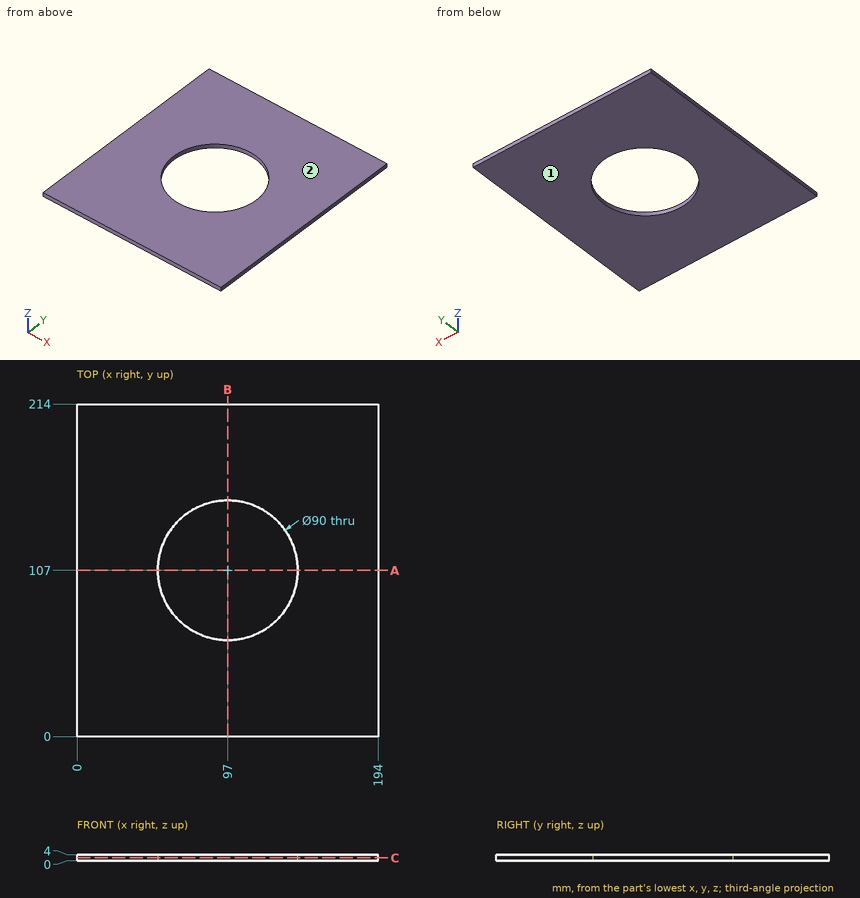
Can you work these out from the drawing? Everything is in mm from the part's minimum corner. Coordinates: 2 decimals unless noted, no trailing zeros. Order: outer loops, then holes, each group sorted by start corner. A loop starts at its lowest first (then second) coordinate and runs counter-clockwise, first axis right, second up. Notation, with made-up numbers: M -6.75,34.5 L 26.25,34.5 A9 ccw 26.25,46.5 Z; hole C 66.25,-26.5 d6. An arc over 180 degrees is marked long. Answer as CSV lines item,"result". Start each with the question number.
1. I want a section at B-B, the plane x = 97. Write out the boundary of the cut face in (y, z), and give its area (3 significant figures).
2. For pin 1 (6 mm diameter, centred on x = 108.5, y = 69.5, fed in from +Z), with a flat end and sliding along its axis, tell me the tip position at first contact or that it passes through.
3. We'd pull the mould along Z, two halves only. Please class the marked faces 1 and 2: released by +Z, released by -Z, zero draft, split by the parting line, or undercut.
4. I want a section at A-A, the plane y = 107. Write out the boundary of the cut face in (x, z), and give its area (3 significant figures).
5. I need wall thicknesses on line 1 (X direction, y = 107, z = 3); line 2 (Y direction, x = 97, z = 0.9); line 3 (Y direction, x = 70.5, z = 3.5). Which ranges of each line are inside material? Lowest first, please. Write a range as [from, to].
6. I want a section at C-C, the plane z = 1.9. Write out the boundary of the cut face in (x, y).
Recorded:
1,outline,"M 0,0 L 62,0 L 62,4 L 0,4 Z; M 152,0 L 214,0 L 214,4 L 152,4 Z"
1,area,"496 mm2"
2,pin 1,"passes through"
3,face 1,"released by -Z"
3,face 2,"released by +Z"
4,outline,"M 0,0 L 52,0 L 52,4 L 0,4 Z; M 142,0 L 194,0 L 194,4 L 142,4 Z"
4,area,"416 mm2"
5,line 1,"x = [0, 52], [142, 194]"
5,line 2,"y = [0, 62], [152, 214]"
5,line 3,"y = [0, 70.63], [143.37, 214]"
6,outline,"M 0,0 L 194,0 L 194,214 L 0,214 Z; hole C 97,107 d90"
